Can you work these out from the model? Positions are in its coordinate system, mm. Face numbers are marked on the shaded views. A direction names the side the tool comes from. Coordinates: 2 decimals unless noted, no trailing zeros. Order: outer loops, then holes, each group sorted by start corner. A loop starts at its lowest first (then second) coordinate and runs counter-clockwise, first axis right, second up. Notation, with made-up numbers: (73, -28.5) - (91, -28.5) arc R20 cw to (91, 7.5) - close; hole circle Ø4 at (68, -8). An arc over 180 degrees is marked (long way). Use a Markdown table: item, result. Add a question column.
(1) I want a section at C-C (y = -15.5). List the corners of the cut face in (x, z) for me, and give its area (3 significant figures).
(2) On a 3-axis mill with a long thin cutter (end or side, diameter ignored), from which of +Z, -Z, +X, -X, +Y, -Y can I reach the whole of each face in a straight line? I mean the marked faces 5, 6, 7, 8 and 9. Say none if no direction works.
(3) If I drill on L1, parallel to Z at x = 30.5, y = -44; L2, parallel to Z at x = 96, y = -27.5; L3, parallel to X at y = -9, z = -62, over which ranges is the centre line in solid material (lowest first)? Write a range as [from, to].
(4) I want a section at A-A (y = -67). List the corners of the cut face in (x, z) for me, and give its area (3 significant figures).
(5) For pin 1 Ø1 at (x, y) = (122, -53.5) entering from +Z; pin 2 Ø8 at (y, z) = (-27.5, -41.5) entering from +X; pin 3 Ø10 at (x, y) = (100.38, -37.13) entering from +Z; pin 4 Ø7.5 at (x, y) = (60, -10) entering from +Z, each with a flat end and sliding along its axis, tell me the tip position at first contact or that it passes through.
(6) I want a section at D-D (z = -31). List the corners of the cut face in (x, y) for me.
(7) I want a section at B-B (x = 25.4). List the corners of the cut face in (y, z) for me, and give its area (3 significant figures).
(8) We'd pull the mould along Z, two halves only. Please class the marked faces 1, 2, 3 and 4: pulls with the +Z half, pulls with the -Z half, needs draft (parallel to the pull), parting line crosses it, or undercut.
```python
from build123d import *

# Parameters (mm, degrees)
F0_W      = 177.8
F0_H      = 88.9
F1_DEPTH  = 76.2
F2_W      = 50.8
F2_H      = 25.4
F3_DEPTH  = 76.2
F4_DEPTH  = 76.2
F5_DEPTH  = 76.2
F6_DEPTH  = 50.8
F7_DEPTH  = 50.8
F8_R      = 6.35
F9_DEPTH  = 25.4
F11_DEPTH = 25.4
F12_DEPTH = 25.4
F13_R     = 6.35
F14_DEPTH = 25.4
F15_R     = 6.35
F16_DEPTH = 50.8
F17_R     = 6.35
F18_DEPTH = 76.2


with BuildPart() as f1:
    # F0 (on Front) → F1 (new body)
    with BuildSketch(Plane.XZ):
        with Locations((88.9, -44.45)):
            Rectangle(F0_W, F0_H)
    extrude(amount=F1_DEPTH)

    # F2 (on face) → F3 (join)
    with BuildSketch(Plane.XZ.offset(76.2)):
        with Locations((25.4, -12.7)):
            Rectangle(F2_W, F2_H)
        Polygon((0, -63.5), (0, -88.9), (177.8, -88.9), (177.8, -63.5), (76.2, -63.5), align=None)
        Polygon((0, -25.4), (0, -63.5), (76.2, -63.5), (76.2, -38.1), (50.8, -38.1), (50.8, -25.4), align=None)
    extrude(amount=-F3_DEPTH)

    # F2 (on face) → F4 (join)
    with BuildSketch(Plane.XZ.offset(76.2)):
        with Locations((25.4, -12.7)):
            Rectangle(F2_W, F2_H)
        Polygon((0, -25.4), (0, -63.5), (76.2, -63.5), (76.2, -38.1), (50.8, -38.1), (50.8, -25.4), align=None)
        Polygon((0, -63.5), (0, -88.9), (177.8, -88.9), (177.8, -63.5), (76.2, -63.5), align=None)
    extrude(amount=-F4_DEPTH)

    # F2 (on face) → F5 (cut)
    with BuildSketch(Plane.XZ.offset(76.2)):
        Polygon((76.2, -38.1), (76.2, -63.5), (177.8, -63.5), (177.8, 0), (50.8, 0), (50.8, -25.4), (50.8, -38.1), align=None)
    extrude(amount=-F5_DEPTH, mode=Mode.SUBTRACT)

    # F2 (on face) → F6 (join)
    with BuildSketch(Plane.XZ.offset(76.2)):
        Polygon((0, -25.4), (0, -63.5), (76.2, -63.5), (76.2, -38.1), (50.8, -38.1), (50.8, -25.4), align=None)
    extrude(amount=-F6_DEPTH)

    # F2 (on face) → F7 (cut)
    with BuildSketch(Plane.XZ.offset(76.2)):
        Polygon((0, -25.4), (0, -63.5), (76.2, -63.5), (76.2, -38.1), (50.8, -38.1), (50.8, -25.4), align=None)
    extrude(amount=-F7_DEPTH, mode=Mode.SUBTRACT)

    # F8 (on Top) → F9 (join)
    with BuildSketch(Plane.XY):
        with Locations((25.4, -50.079788)):
            Circle(F8_R)
    extrude(amount=-F9_DEPTH)

    # F10 (on Top) → F11 (cut)
    with BuildSketch(Plane.XY):
        with BuildLine():
            ThreePointArc((19.05, -50.879826), (25.4, -57.229826), (31.75, -50.879826))
            ThreePointArc((31.75, -50.879826), (25.4, -44.529826), (19.05, -50.879826))
        make_face()
    extrude(amount=-F11_DEPTH, mode=Mode.SUBTRACT)

    # F10 (on Top) → F12 (cut)
    with BuildSketch(Plane.XY):
        with BuildLine():
            ThreePointArc((19.05, -50.879826), (25.4, -57.229826), (31.75, -50.879826))
            ThreePointArc((31.75, -50.879826), (25.4, -44.529826), (19.05, -50.879826))
        make_face()
    extrude(amount=-F12_DEPTH, mode=Mode.SUBTRACT)

    # F13 (on Top) → F14 (cut)
    with BuildSketch(Plane.XY):
        with Locations((139.137983, -37.799459)):
            Circle(F13_R)
        with Locations((101.160564, -37.799459)):
            Circle(F13_R)
    extrude(amount=-F14_DEPTH, mode=Mode.SUBTRACT)

    # F15 (on face) → F16 (cut)
    with BuildSketch(Plane.XY.offset(-63.5)):
        with Locations((100.378424, -37.129913)):
            Circle(F15_R)
    extrude(amount=-F16_DEPTH, mode=Mode.SUBTRACT)

    # F17 (on Top) → F18 (cut)
    with BuildSketch(Plane.XY):
        with Locations((136.710018, -37.558652)):
            Circle(F17_R)
    extrude(amount=-F18_DEPTH, mode=Mode.SUBTRACT)


solid = f1.part
```
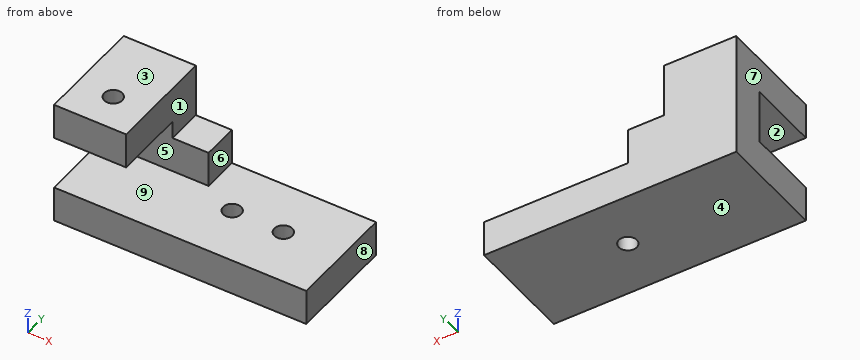
Answers follow:
| question | item | result |
|---|---|---|
| 1 | outline | (0, -88.9) - (177.8, -88.9) - (177.8, -63.5) - (76.2, -63.5) - (76.2, -38.1) - (50.8, -38.1) - (50.8, 0) - (0, 0) - close |
| 1 | area | 8,390 mm² |
| 2 | face 5 | +X, -X, -Y |
| 2 | face 6 | +Z, +X, +Y, -Y |
| 2 | face 7 | +Z, -Z, -X, +Y, -Y |
| 2 | face 8 | +Z, -Z, +X, +Y, -Y |
| 2 | face 9 | +X, -Y |
| 3 | L1 | z = [-88.9, -63.5], [-25.4, 0] |
| 3 | L2 | z = [-88.9, -63.5] |
| 3 | L3 | x = [0, 76.2] |
| 4 | outline | (0, -88.9) - (177.8, -88.9) - (177.8, -63.5) - (0, -63.5) - close; (0, -25.4) - (50.8, -25.4) - (50.8, 0) - (0, 0) - close |
| 4 | area | 5,810 mm² |
| 5 | pin 1 | stops at z = -63.5 |
| 5 | pin 2 | stops at x = 76.2 |
| 5 | pin 3 | passes through |
| 5 | pin 4 | stops at z = -38.1 |
| 6 | outline | (0, -25.4) - (50.8, -25.4) - (50.8, 0) - (0, 0) - close |
| 7 | outline | (-76.2, -88.9) - (0, -88.9) - (0, 0) - (-44.53, 0) - (-44.53, -25.4) - (-25.4, -25.4) - (-25.4, -63.5) - (-76.2, -63.5) - close; (-76.2, -25.4) - (-57.23, -25.4) - (-57.23, 0) - (-76.2, 0) - close |
| 7 | area | 4,520 mm² |
| 8 | face 1 | needs draft |
| 8 | face 2 | undercut |
| 8 | face 3 | pulls with the +Z half |
| 8 | face 4 | pulls with the -Z half |
